Geometry check sheet. Reference: drawing and pictorial views, mm from the part's lowest x, y, z. A direction names the side the tool comes from. Give positions to 0.01 mm unless a question says otherwise; leave off trailing zeros. Loops run counter-clockwise (first coordinate to the right, second up) from the corner with the lowest first, then second, coordinate; pieces in that order, holes last. Notation, with made-up numbers: (-19.5, 60) -> (-9.5, 60) arc R30 ccw to (-9.5, 97) -> close; hole circle Ø3 at (18, 11). An arc over 180 degrees is marked (long way). Write each question's results on one line, items separated by ' | '. Start each with the question number.
1. Cross-section at C-C on x = 5.5. Record the boundary of the cut face in (y, z), and give its area (3 significant figures).
2. Cross-section at D-D on y = 5. Record the boundary of the cut face in (x, z), and give its area (3 significant figures).
3. Cross-section at A-A on z = 5.5. Record the boundary of the cut face in (x, y).
4. Mould release check, pull along X, two halves, no side actions. Record for the marked faces 1, 2 and 3: +X half, -X half, draft (parallel to the pull), parting line (faces both ways), or undercut.
5. Cross-section at B-B on y = 7.5. Record the boundary of the cut face in (x, z).
6. Gauge pin test, flat ends, axial feed: pin 1 Ø1.6 at (x, z) = (5, 2) entering from +Y (1 decimal); pin 2 Ø6 at (y, z) = (6, 9) entering from +X; pin 3 Ø2.5 at (y, z) = (9, 10) entering from +X; pin 4 Ø5 at (x, y) = (5, 7.5) entering from -Z. Record the tip position at first contact, or that the pin passes through.
7. Material ranges on L1, parallel to X at y = 6.25, z = 5.5; L2, parallel to X at y = 10.5, z = 1.25; L3, parallel to Y at x = 5.75, z = 9.75, recorded low to high. Write a range as from..to.
8. Tool access check on the marked faces 4, 5 and 6. Record the directions out of +Z, -Z, +X, -X, +Y, -Y that give a thin tool (end or side, any length) a straight path to the whole face; none if there is none.
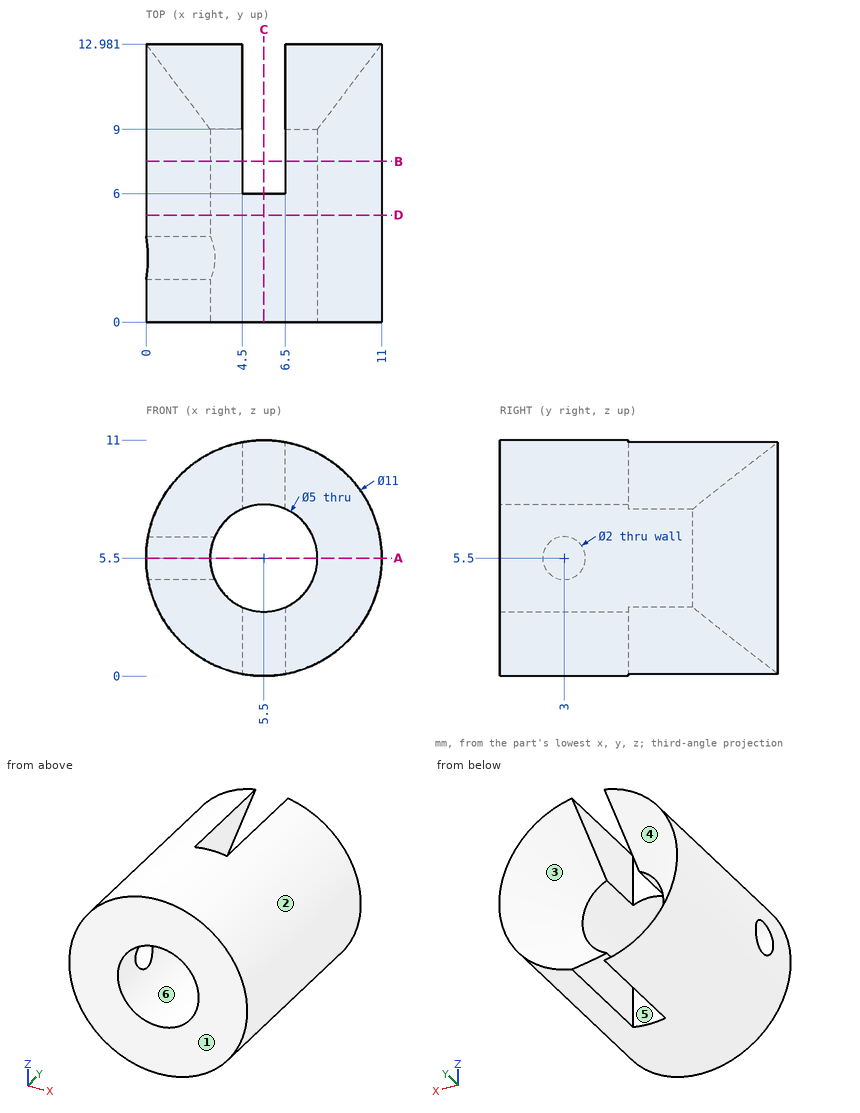
Geometry says:
1) outline: (0, 0) -> (6, 0) -> (6, 3) -> (0, 3) -> close; (0, 8) -> (6, 8) -> (6, 11) -> (0, 11) -> close | area: 36.0 mm^2
2) outline: circle Ø11 at (5.5, 5.5); hole circle Ø5 at (5.5, 5.5) | area: 75.4 mm^2
3) outline: (0, 0) -> (3, 0) -> (3, 2) -> (0, 2) -> close; (0, 4) -> (3, 4) -> (3, 9) -> (0, 12.98) -> close; (8, 0) -> (11, 0) -> (11, 12.98) -> (8, 9) -> close
4) face 1: draft | face 2: parting line | face 3: undercut
5) outline: (4.5, 0.09) -> (4.5, 3.21) arc R2.5 cw to (4.5, 7.79) -> (4.5, 10.91) arc R5.5 ccw to start; (6.5, 0.09) arc R5.5 ccw to (6.5, 10.91) -> (6.5, 7.79) arc R2.5 cw to (6.5, 3.21) -> close
6) pin 1: y = 11.3 | pin 2: x = 10.98 | pin 3: x = 9.94 | pin 4: z = 0
7) L1: 0..3, 8..11 | L2: 2.01..4.5, 6.5..8.99 | L3: 0..6
8) face 4: +Y | face 5: +Z, -Z, +Y | face 6: +Y, -Y
